Could you check a few things on this model? Use its own coordinates, in mm. A direction names the side the tool comes from. Coordinates: 2 decimals unless noted, no trailing zeros. Order: outer loops, then holes, each group sorted by start corner. A loop starts at its lowest first (then second) coordinate and runs counter-clockwise, first axis right, second up. Notation, with made-up numbers: (59, -18) -> (63, -18) arc R21 cw to (63, 2) -> close; hole circle Ø11 at (-29, 14). An arc over 180 degrees is marked (long way). Return JSON: item names as keys, results as strings. Group by question number.
Autodesk Inventor part; units mm, degrees
ref_plane "Work Plane1" through (50.8, 0, 0) normal (1, 0, 0) x (0, 0, -1)
ref_plane "YZ Plane" through (0, 0, 0) normal (1, 0, 0) x (0, 1, 0)
ref_plane "XZ Plane" through (0, 0, 0) normal (0, 1, 0) x (-1, 0, 0)
sketch "Sketch1" plane through (0, 0, 0) normal (1, 0, 0) x (0, 1, 0)
  circle A0 centre (0, 0) radius 88.9
  circle A1 centre (0, 0) radius 92.075
  dimension "d0" = 177.8
  dimension "d1" = 184.15
extrude "Extrusion1" add sketch "Sketch1" along normal blind 101.6
ref_plane "Work Plane1" through (50.8, 0, 0) normal (1, 0, 0) x (0, 0, -1)
sketch "Sketch5" plane through (0, 0, 0) normal (0, 1, 0) x (-1, 0, 0)
  line L0 (20.32, 0) -> (-121.92, 0)
  line L1 (0, -88.9) -> (0, 88.9)
  line L2 (0, 88.9) -> (-101.6, 88.9)
  line L3 (-101.6, 92.075) -> (-101.6, -92.075)
  line L4 (-101.6, -88.9) -> (-101.6, 88.9)
  arc A0 (-101.6, 88.9) -> (0, 88.9) centre (-50.8, 88.9) ccw
  point P0 (0, 0)
  dimension "d23" = 50.8
revolve "Revolution1" add sketch "Sketch5" angle 360 about axis through (-10, 0, 0) along (1, 0, 0) contours A0 L2
sketch "Sketch6" plane through (0, 0, 0) normal (1, 0, 0) x (0, 1, 0)
  circle A0 centre (0, 0) radius 104.775
  circle A1 centre (0, 0) radius 107.95
  dimension "d17" = 215.9
  dimension "d18" = 209.55
extrude "Extrusion3" add sketch "Sketch6" along normal blind 101.6 and the other way blind 25.4
sketch "Sketch7" plane through (101.6, 0, 0) normal (1, 0, 0) x (0, 0, -1)
  circle A0 centre (0, 0) radius 107.95
  circle A1 centre (0, 0) radius 87.7627
extrude "Extrusion4" add sketch "Sketch7" along normal blind 6.35
fillet "Fillet1" radius 3.175 2 edges at (107.95, 0, 87.7627) (107.95, 0, 107.95)
properties part number "AirBagV1" material "Steel, Alloy"
Q1. I want a section at D-D on x = 81. State how many separate pieces and enclosed holes the cut face has, and give its area (3 significant figures).
Q2. We'd pull the mould along Z, two halves only. Please class faces 4 (the cylindrical face through (50.089, -73.068, 56.026)), 5 (the flat face through (107.95, 86, 32)), 6 (the cylindrical face through (38.776, 100.195, -40.177)), 7 (the flat face through (0, -48.2, 75.5)): pulls with the +Z half, pulls with the -Z half, needs draft (parallel to the pull), parting line crosses it, or undercut.
Q3. I want a section at C-C on x = 16.5. Please give me the cut outline in (y, z) (3 decimals).
Q4. I want a section at A-A on y = 0. Please give me the cut outline in (x, z) (3 decimals).
Q5. I need wall thicknesses on line 1 along Z through (x, y) = (16.5, 84); line 2 along Y through (x, z) = (52.5, 57); line 3 along Z through (x, y) = (53.5, -69). Which ranges of each line are inside material? Lowest first, please. Write a range as from..to.
Q6. I'm going to push flat-ended pins straight in: pin 1 Ø2 at (x, z) = (20.5, 36) entering from +Y; pin 2 Ø5 at (x, z) = (78, -37.5) entering from -Y; pin 3 Ø3 at (y, z) = (-80.5, -34) entering from +X. Where does each tip first touch, or does it pass through?
Q7. On a 3-axis mill with a long thin cutter (end or side, diameter ignored), from which of +Z, -Z, +X, -X, +Y, -Y can I reach the whole of each face in a straight line? I mean faces 1 (the cylindrical face through (38.989, -22.713, -102.283)), 2 (the cylindrical face through (103.165, -3.859, 87.678)), 3 (the flat face through (-25.4, -56.5, 88.5)). Say none if no direction works.
Response values:
{
 "1": {"separate pieces": "2", "enclosed holes": "2", "area": "21,500 mm²"},
 "2": {"face 4": "undercut", "face 5": "needs draft", "face 6": "parting line crosses it", "face 7": "undercut"},
 "3": {"outline": "circle Ø215.9 at (0, 0); circle Ø184.15 at (0, 0); hole circle Ø209.55 at (0, 0); hole circle Ø102.856 at (0, 0)"},
 "4": {"outline": "(-25.4, -107.95) -> (104.775, -107.95) arc R3.175 ccw to (107.95, -104.775) -> (107.95, -90.938) arc R3.175 ccw to (104.775, -87.763) -> (101.6, -87.763) -> (101.6, -88.9) arc R50.8 ccw to (0, -88.9) -> (0, -92.075) -> (101.6, -92.075) -> (101.6, -104.775) -> (-25.4, -104.775) -> close; (-25.4, 104.775) -> (101.6, 104.775) -> (101.6, 92.075) -> (0, 92.075) -> (0, 88.9) arc R50.8 ccw to (101.6, 88.9) -> (101.6, 87.763) -> (104.775, 87.763) arc R3.175 ccw to (107.95, 90.938) -> (107.95, 104.775) arc R3.175 ccw to (104.775, 107.95) -> (-25.4, 107.95) -> close"},
 "5": {"line 1": "z = -67.8..-62.62, -37.71..37.71, 62.62..67.8", "line 2": "y = -91.67..-87.91, -72.31..72.31, 87.91..91.67", "line 3": "z = -83.02..-78.85, -60.97..60.97, 78.85..83.02"},
 "6": {"pin 1": "stops at y = 102.12", "pin 2": "stops at y = -102.12", "pin 3": "stops at x = 107.2"},
 "7": {"face 1": "-X", "face 2": "+X", "face 3": "+Z, -Z, -X, +Y, -Y"}
}
